Can you work these out from the model? Positions are in its coordinate system, mm. A direction names the side the tool comes from. Coordinates: 2 decimals unless noted, no trailing zeros. Order: outer loops, then holes, each group sorted by start corner. A loop starts at its lowest first (then second) coordinate and runs counter-clockwise, first axis right, second up. Notation, with made-up numbers: (-28, 64) -> (17, 64) arc R21 cw to (17, 85) -> close; hole circle Ø9 at (32, 36). An arc over 180 degrees is marked (long way). Answer in a Markdown table with one row per item. Add a question column.
1. Imagine slicing it at B-B on z = 0. Write out the boundary of the cut face in (x, y).
2. Imagine slicing it at A-A on x = 0. Write out the boundary of the cut face in (y, z), plus the area to 3 significant figures.
3. On a 3-axis mill with a long thin cutter (end or side, diameter ignored), from which of +Z, -Z, +X, -X, +Y, -Y can I reach the whole of each face in a straight line? I mean faces 1 (the face through (0, 9, -23)), 2 (the face through (17, 13, -18)), 3 (the face through (7.5, 6, -23)). Say none if no direction works.
4. If I drill on line 1 along Y through (x, z) = (-8, 15); line 2 along Z through (x, y) = (-9.5, 16.5); line 3 along X through (y, z) = (8, -23.5), over which ranges is the centre line in solid material (lowest first)? Write a range as [from, to].
5. We'd pull the mould along Z, two halves only. Please class faces 4 (the face through (18, 13, 17)), 5 (the face through (0, 45, 0)), 6 (the face through (16, 18.5, -16)), 7 (the face through (-2, 23, 2)): pulls with the +Z half, pulls with the -Z half, needs draft (parallel to the pull), parting line crosses it, or undercut.
6. Imagine slicing it at D-D on z = -5. Write out the boundary of the cut face in (x, y).
7. Will these pins go through, and if not, where does the flat tip stop? pin 1 (7 mm diameter, centred on x = 3.5, y = 10, fed in from -Z); pin 2 (5.5 mm diameter, centred on y = 7, z = -24.5, fed in from -X); pin 3 (0.9 mm diameter, centred on x = -16, z = -16, fed in from +Y); pin 4 (3.5 mm diameter, centred on x = -16, z = 15, fed in from +Y).
8. Imagine slicing it at C-C on y = 37. Write out the boundary of the cut face in (x, z), plus the area to 3 significant figures.
from build123d import *

# Parameters (mm, degrees)
BOSS_EXTRUDE1_DEPTH = 9
BOSS_EXTRUDE2_DEPTH = 9
BOSS_EXTRUDE3_DEPTH = 5
SKETCH5_R           = 11
SKETCH5_R_2         = 9
BOSS_EXTRUDE4_DEPTH = 2
SKETCH6_R           = 2.5
BOSS_EXTRUDE5_DEPTH = 22
SKETCH7_R           = 1.5
CUT_EXTRUDE1_DEPTH  = 4.5
SKETCH9_W           = 15
SKETCH9_H           = 5
BOSS_EXTRUDE6_DEPTH = 5


with BuildPart() as part:
    # Sketch2 → Boss-Extrude1 (new body)
    with BuildSketch(Plane(origin=(0, 0, 0), x_dir=(1, 0, 0), z_dir=(0, 1, 0))):
        with BuildLine():
            Line((-18, 21), (18, 21))
            ThreePointArc((18, 21), (20.121320344, 20.121320344), (21, 18))
            Line((21, 18), (21, -18))
            ThreePointArc((21, -18), (20.121320344, -20.121320344), (18, -21))
            Line((18, -21), (-18, -21))
            ThreePointArc((-18, -21), (-20.121320344, -20.121320344), (-21, -18))
            Line((-21, -18), (-21, 18))
            ThreePointArc((-21, 18), (-20.121320344, 20.121320344), (-18, 21))
        make_face()
    extrude(amount=BOSS_EXTRUDE1_DEPTH)

    # Sketch3 → Boss-Extrude2 (add)
    with BuildSketch(Plane(origin=(0, 9, 0), x_dir=(1, 0, 0), z_dir=(0, 1, 0))):
        Polygon((-21, 14), (-14, 21), (14, 21), (21, 14), (21, -14), (14, -21), (-14, -21), (-21, -14), align=None)
    extrude(amount=BOSS_EXTRUDE2_DEPTH)

    # Sketch4 → Boss-Extrude3 (add)
    with BuildSketch(Plane(origin=(0, 18, 0), x_dir=(1, 0, 0), z_dir=(0, 1, 0))):
        with BuildLine():
            Line((-18, 21), (18, 21))
            ThreePointArc((18, 21), (20.121320344, 20.121320344), (21, 18))
            Line((21, 18), (21, -18))
            ThreePointArc((21, -18), (20.121320344, -20.121320344), (18, -21))
            Line((18, -21), (-18, -21))
            ThreePointArc((-18, -21), (-20.121320344, -20.121320344), (-21, -18))
            Line((-21, -18), (-21, 18))
            ThreePointArc((-21, 18), (-20.121320344, 20.121320344), (-18, 21))
        make_face()
    extrude(amount=BOSS_EXTRUDE3_DEPTH)

    # Sketch5 → Boss-Extrude4 (add)
    with BuildSketch(Plane(origin=(0, 23, 0), x_dir=(1, 0, 0), z_dir=(0, 1, 0))):
        with Locations(Location((0, 0, 0), (0, 0, 270))):
            Circle(SKETCH5_R)
        with Locations(Location((0, 0, 0), (0, 0, 270))):
            Circle(SKETCH5_R_2, mode=Mode.SUBTRACT)
    extrude(amount=BOSS_EXTRUDE4_DEPTH)

    # Sketch6 → Boss-Extrude5 (add)
    with BuildSketch(Plane(origin=(0, 23, 0), x_dir=(1, 0, 0), z_dir=(0, 1, 0))):
        with Locations(Location((0, 0, 0), (0, 0, 270))):
            Circle(SKETCH6_R)
    extrude(amount=BOSS_EXTRUDE5_DEPTH)

    # Sketch7 → Cut-Extrude1 (cut)
    with BuildSketch(Plane(origin=(0, 23, 0), x_dir=(1, 0, 0), z_dir=(0, 1, 0))):
        with Locations(Location((-15.5, 15.5, 0), (0, 0, 270))):
            Circle(SKETCH7_R)
        with Locations(Location((15.505550331, 15.61144176, 0), (0, 0, 270))):
            Circle(SKETCH7_R)
        with Locations(Location((15.732618971, -15.912931541, 0), (0, 0, 270))):
            Circle(SKETCH7_R)
        with Locations(Location((-15.494867745, -15.663236697, 0), (0, 0, 270))):
            Circle(SKETCH7_R)
    extrude(amount=-CUT_EXTRUDE1_DEPTH, mode=Mode.SUBTRACT)

    # Sketch9 → Boss-Extrude6 (add)
    with BuildSketch(Plane(origin=(0, 0, -21), x_dir=(-1, 0, 0), z_dir=(0, 0, -1))):
        with Locations((0, 6.5)):
            Rectangle(SKETCH9_W, SKETCH9_H)
    extrude(amount=BOSS_EXTRUDE6_DEPTH)


solid = part.part
Answers follow:
| question | item | result |
|---|---|---|
| 1 | outline | (-21, 0) -> (21, 0) -> (21, 23) -> (11, 23) -> (11, 25) -> (9, 25) -> (9, 23) -> (2.5, 23) -> (2.5, 45) -> (-2.5, 45) -> (-2.5, 23) -> (-9, 23) -> (-9, 25) -> (-11, 25) -> (-11, 23) -> (-21, 23) -> close |
| 2 | outline | (0, -21) -> (4, -21) -> (4, -26) -> (9, -26) -> (9, -21) -> (23, -21) -> (23, -11) -> (25, -11) -> (25, -9) -> (23, -9) -> (23, -2.5) -> (45, -2.5) -> (45, 2.5) -> (23, 2.5) -> (23, 9) -> (25, 9) -> (25, 11) -> (23, 11) -> (23, 21) -> (0, 21) -> close |
| 2 | area | 1,110 mm² |
| 3 | face 1 | -Z, +X, -X, +Y |
| 3 | face 2 | -Z, +X |
| 3 | face 3 | -Z, +X, +Y, -Y |
| 4 | line 1 | y = [0, 23] |
| 4 | line 2 | z = [-21, 21] |
| 4 | line 3 | x = [-7.5, 7.5] |
| 5 | face 4 | pulls with the +Z half |
| 5 | face 5 | needs draft |
| 5 | face 6 | undercut |
| 5 | face 7 | undercut |
| 6 | outline | (-21, 0) -> (21, 0) -> (21, 23) -> (9.8, 23) -> (9.8, 25) -> (7.48, 25) -> (7.48, 23) -> (-7.48, 23) -> (-7.48, 25) -> (-9.8, 25) -> (-9.8, 23) -> (-21, 23) -> close |
| 7 | pin 1 | stops at z = -26 |
| 7 | pin 2 | stops at x = -7.5 |
| 7 | pin 3 | stops at y = 18.5 |
| 7 | pin 4 | stops at y = 23 |
| 8 | outline | circle Ø5 at (0, 0) |
| 8 | area | 19.6 mm² |
